from build123d import *

# Parameters (mm, degrees)
BOSS_EXTRUDE1_DEPTH = 6.35
SKETCH2_R           = 1.25
CUT_EXTRUDE1_DEPTH  = 7.35


with BuildPart() as part:
    # Sketch1 → Boss-Extrude1 (new body)
    with BuildSketch(Plane.XY):
        Polygon((0, -6.35), (6.35, -6.35), (6.35, 0), (6.8453, 0), (6.8453, 10.795), (12.7, 10.795), (12.7, 29.845), (6.8453, 29.845), (6.8453, 60.325), (6.35, 60.325), (6.35, 66.675), (0, 66.675), (0, 60.325), (-0.4953, 60.325), (-0.4953, 29.845), (-6.35, 29.845), (-6.35, 10.795), (-0.4953, 10.795), (-0.4953, 0), (0, 0), align=None)
    extrude(amount=BOSS_EXTRUDE1_DEPTH)

    # Sketch2 → Cut-Extrude1 (cut, through all)
    with BuildSketch(Plane.XY.offset(6.35)):
        with Locations((-3.42265, 20.32)):
            Circle(SKETCH2_R)
        with Locations((9.77265, 20.32)):
            Circle(SKETCH2_R)
    extrude(amount=-CUT_EXTRUDE1_DEPTH, mode=Mode.SUBTRACT)


solid = part.part
Could you check a few things on this model? Use its own coordinates, in mm. A direction names the side the tool comes from. Give positions to 0.01 mm unless a question says otherwise; leave off trailing zeros. Order: outer loops, then holes, each group sorted by start corner. A loop starts at its lowest first (then second) coordinate and runs counter-clockwise, first axis right, second up.
1. For pin 1 (2 mm diameter, centred on x = 9.77, y = 20.32, fed in from +Z); pin 2 (1.8 mm diameter, centred on x = -2, z = 1.5, fed in from +Y) (3 decimals); pin 3 (3 mm diameter, centred on y = 39.5, z = 3, fed in from -X); pin 4 (0.5 mm diameter, centred on x = -0.5, z = 4.5, fed in from +Y) (3 decimals), each with a flat end and sliding along its axis, tell me the tip position at first contact or that it passes through.
Answers below:
pin 1: passes through
pin 2: stops at y = 29.845
pin 3: stops at x = -0.5
pin 4: stops at y = 60.325
2. Suppose I cut it at B-B (z = 1). Write out the boundary of the cut face in (x, y) (3 decimals).
Answers below:
outline: (-6.35, 10.795) - (-0.495, 10.795) - (-0.495, 0) - (0, 0) - (0, -6.35) - (6.35, -6.35) - (6.35, 0) - (6.845, 0) - (6.845, 10.795) - (12.7, 10.795) - (12.7, 29.845) - (6.845, 29.845) - (6.845, 60.325) - (6.35, 60.325) - (6.35, 66.675) - (0, 66.675) - (0, 60.325) - (-0.495, 60.325) - (-0.495, 29.845) - (-6.35, 29.845) - close; hole circle Ø2.5 at (-3.423, 20.32); hole circle Ø2.5 at (9.773, 20.32)
3. Which directions (+Z, -Z, +X, -X, +Y, -Y) give clear straight access to the entire face, cutting with the end or side of a thin tool? Please do faces 1 (the flat face through (-3, 10.795, 3)), 2 (the flat face through (-3, 29.845, 3)), 3 (the flat face through (6.845, 5, 3)).
Answers below:
face 1: +Z, -Z, -X, -Y
face 2: +Z, -Z, -X, +Y
face 3: +Z, -Z, +X, -Y
4. Suppose I cut it at A-A (y = 20.32). Write out the boundary of the cut face in (x, z), plus the area to 3 significant figures.
Answers below:
outline: (-6.35, 0) - (-4.67, 0) - (-4.67, 6.35) - (-6.35, 6.35) - close; (-2.17, 0) - (8.52, 0) - (8.52, 6.35) - (-2.17, 6.35) - close; (11.02, 0) - (12.7, 0) - (12.7, 6.35) - (11.02, 6.35) - close
area: 89.2 mm2
5. Suppose I cut it at D-D (y = 58). Write out the boundary of the cut face in (x, z), plus the area to 3 significant figures.
Answers below:
outline: (-0.5, 0) - (6.85, 0) - (6.85, 6.35) - (-0.5, 6.35) - close
area: 46.6 mm2
6. Thinking about a two-plate mould opening in X: for faces 4 (the flat face through (3, 31, 6.35)), 5 (the flat face through (6.845, 45, 3)), 6 (the cylindrical face through (-2.27, 19.84, 3.22)), which applies, +X half, -X half, draft (parallel to the pull), parting line (faces both ways), or undercut?
Answers below:
face 4: draft
face 5: +X half
face 6: undercut
7. I need wall thicknesses on L1, parallel to Y at x = 7.25, z = 2 (3 decimals); L2, parallel to Y at x = 9.5, z = 6.25 (3 decimals); L3, parallel to X at y = 35.5, z = 3.75. Which ranges of each line are inside material? Lowest first, please.
Answers below:
L1: y = 10.795 to 29.845
L2: y = 10.795 to 19.1, 21.54 to 29.845
L3: x = -0.5 to 6.85
8. Suppose I cut it at C-C (x = 9.5). Write out the boundary of the cut face in (y, z) (3 decimals), plus the area to 3 significant figures.
Answers below:
outline: (10.795, 0) - (19.1, 0) - (19.1, 6.35) - (10.795, 6.35) - close; (21.54, 0) - (29.845, 0) - (29.845, 6.35) - (21.54, 6.35) - close
area: 105 mm2
